Geometry check sheet. Reference: the model listing, model coordinates, mm. Give positions to 0.01 mm unless a question says otherwise; leave off trailing zeros. Loops run counter-clockwise (first coordinate to the right, second up) from the corner with the lowest first, then second, coordinate; pieces in that order, holes last. Notation, with made-up numbers: (7.25, 27) -> (38.25, 27) arc R20 ccw to (38.25, 52) -> close; hole circle Ø1 at (-2, 8.5). An arc over 180 degrees is marked (long way). Write item = value, one per line.
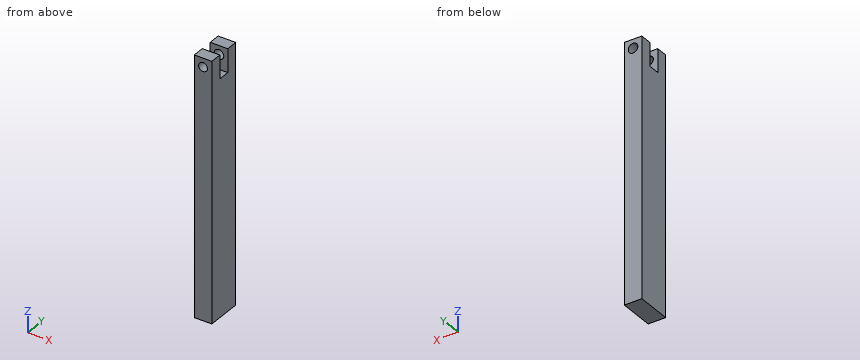
Autodesk Inventor part; units mm, degrees
ref_plane "YZ Plane" through (0, 0, 0) normal (1, 0, 0) x (0, 1, 0)
ref_plane "XZ Plane" through (0, 0, 0) normal (0, 1, 0) x (-1, 0, 0)
ref_plane "XY Plane" through (0, 0, 0) normal (0, 0, 1) x (1, 0, 0)
sketch "Sketch1" plane through (0, 0, 0) normal (1, 0, 0) x (0, 1, 0)
  line L0 (-9.525, -69.85) -> (9.525, -69.85)
  line L1 (9.525, -69.85) -> (9.525, 69.85)
  line L2 (9.525, 69.85) -> (-9.525, 69.85)
  line L3 (-9.525, 69.85) -> (-9.525, -69.85)
  line L4 (-9.525, -69.85) -> (9.525, 69.85) construction
  line L5 (9.525, -69.85) -> (-9.525, 69.85) construction
  point P0 (0, 0)
  dimension "d0" = 19.05
  dimension "d1" = 139.7
extrude "Extrusion1" add sketch "Sketch1" along normal mid plane 9.525
sketch "Sketch2" plane through (4.7625, 0, 0) normal (1, 0, 0) x (0, 0, -1)
  line L0 (-82.55, -3.175) -> (-57.15, -3.175)
  line L1 (-57.15, -3.175) -> (-57.15, 3.175)
  line L2 (-57.15, 3.175) -> (-82.55, 3.175)
  line L3 (-82.55, 3.175) -> (-82.55, -3.175)
  line L4 (-69.85, 9.525) -> (-69.85, -9.525)
  line L5 (-82.55, -3.175) -> (-57.15, 3.175) construction
  line L6 (-57.15, -3.175) -> (-82.55, 3.175) construction
  point P0 (0, 0)
  point P1 (-69.85, 0)
  point P2 (-69.85, 3.175)
  point P3 (-69.85, -3.175)
  dimension "d4" = 6.35
  dimension "d5" = 12.7
extrude "Extrusion2" cut sketch "Sketch2" against normal blind 25.4 contours L4 L2 L1 L0
sketch "Sketch3" plane through (-4.7625, 9.525, 69.85) normal (0, 1, 0) x (1, 0, 0)
  line L0 (9.525, 0) -> (0, 0)
  circle A0 centre (4.7625, 4.7625) radius 2.6035
  point P0 (4.7625, 69.85)
  point P1 (4.7625, 0)
  dimension "d8" = 5.207
  dimension "d9" = 4.7625
extrude "Extrusion3" cut sketch "Sketch3" against normal blind 6.35
sketch "Sketch4" plane through (-4.7625, 9.525, 69.85) normal (0, 1, 0) x (1, 0, 0)
  circle A0 centre (4.7625, 4.7625) radius 2.6035
  circle A1 centre (4.7625, 4.7625) radius 2.3813
  point P0 (4.7625, 69.85)
  dimension "d12" = 4.7625
extrude "Extrusion4" cut sketch "Sketch4" against normal blind 25.4 contours A1
properties part number "ShortBraillePlunger"
Item 1: Thickness scan on L1, parallel to Z at x = 0, y = -4.5; L2, parallel to Y at x = -3.75, z = 59.5 (3 decimals); L3, parallel to Z at x = 0, y = 7. Record the ranges inside material, lowest first. Write a range as [from, to].
Answer:
L1 = [-69.85, 62.71], [67.47, 69.85]
L2 = [-9.525, -3.175], [3.175, 9.525]
L3 = [-69.85, 62.48], [67.69, 69.85]
Item 2: Gauge pin test, flat end, axial feed: pin 1 (4 mm diameter, centred on x = -2, y = -1, fed in from +Z). Record the tip position at first contact, or that the pin passes through.
Answer:
pin_1 = 57.15
Item 3: Section check B-B, the plane z = 61. Record the cut outline in (x, y) (1 decimal).
Answer:
outline = (-4.8, -9.5) -> (4.8, -9.5) -> (4.8, -3.2) -> (-4.8, -3.2) -> close; (-4.8, 3.2) -> (4.8, 3.2) -> (4.8, 9.5) -> (-4.8, 9.5) -> close
Item 4: Section check A-A, the plane x = 0. Record the cut outline in (y, z) (3 decimals), plus the area to 3 significant figures.
Answer:
outline = (-9.525, -69.85) -> (9.525, -69.85) -> (9.525, 62.484) -> (3.175, 62.484) -> (3.175, 57.15) -> (-3.175, 57.15) -> (-3.175, 62.706) -> (-9.525, 62.706) -> close; (-9.525, 67.469) -> (-3.175, 67.469) -> (-3.175, 69.85) -> (-9.525, 69.85) -> close; (3.175, 67.691) -> (9.525, 67.691) -> (9.525, 69.85) -> (3.175, 69.85) -> close
area = 2,520 mm^2
Item 5: Section check C-C, the plane y = 6.75. Record the cut outline in (x, z).
Answer:
outline = (-4.76, -69.85) -> (4.76, -69.85) -> (4.76, 69.85) -> (-4.76, 69.85) -> close; hole circle Ø5.21 at (0, 65.09)
Item 6: Section check D-D, the plane y = -1.25. Record the cut outline in (x, z), plus the area to 3 significant figures.
Answer:
outline = (-4.76, -69.85) -> (4.76, -69.85) -> (4.76, 57.15) -> (-4.76, 57.15) -> close
area = 1,210 mm^2
